Autodesk Inventor part; units mm, degrees
ref_plane "YZ Plane" through (0, 0, 0) normal (1, 0, 0) x (0, 1, 0)
ref_plane "XZ Plane" through (0, 0, 0) normal (0, 1, 0) x (-1, 0, 0)
ref_plane "XY Plane" through (0, 0, 0) normal (0, 0, 1) x (1, 0, 0)
sketch "Boceto1" plane through (0, 0, 0) normal (0, 0, 1) x (1, 0, 0)
  line L0 (-46, -14.91) -> (-46, -35.91)
  line L1 (-44.1, -31.91) -> (-2.9, -31.91)
  line L2 (-1, -35.91) -> (-1, -20.31)
  line L3 (-8.1, 6.6131) -> (-8.1, -14.91)
  line L4 (-44.6, -16.31) -> (-6.4, -16.31)
  line L5 (-2.4, -20.31) -> (-2.4, -30.01)
  line L6 (-2.9, -30.51) -> (-44.1, -30.51)
  line L7 (-44.6, -30.01) -> (-44.6, -16.31)
  arc A0 (-2.4, -20.31) -> (-6.4, -16.31) centre (-6.4, -20.31) ccw
  line L8 (-2.4, -32.41) -> (-2.4, -34.1632)
  line L9 (-3.5, -35.91) -> (-1, -35.91)
  line L10 (-9.5, -14.91) -> (-9.5, 7.7994)
  line L11 (-44.6, -32.41) -> (-44.6, -34.2323)
  line L12 (-43.5, -35.91) -> (-46, -35.91)
  line L13 (-43.5, -35.91) -> (-43.5, -35.4546)
  line L14 (-3.5, -35.91) -> (-3.5, -35.21)
  line L15 (-43.7447, -35.0247) -> (-44.3553, -34.6622)
  line L16 (-3.5, -35.21) -> (-2.6082, -34.5692)
  arc A1 (-2.9, -30.51) -> (-2.4, -30.01) centre (-2.9, -30.01) ccw
  arc A2 (-2.4, -32.41) -> (-2.9, -31.91) centre (-2.9, -32.41) ccw
  arc A3 (-2.6082, -34.5692) -> (-2.4, -34.1632) centre (-2.9, -34.1632) ccw
  arc A4 (-44.6, -30.01) -> (-44.1, -30.51) centre (-44.1, -30.01) ccw
  arc A5 (-44.1, -31.91) -> (-44.6, -32.41) centre (-44.1, -32.41) ccw
  arc A6 (-44.6, -34.2323) -> (-44.3553, -34.6622) centre (-44.1, -34.2323) ccw
  arc A7 (-43.5, -35.4546) -> (-43.7447, -35.0247) centre (-44, -35.4546) ccw
  line L17 (-9.5, 7.7994) -> (-4.75, 8.59)
  line L18 (-4.75, 8.59) -> (0, 7.7994)
  line L19 (-8.1, 6.6131) -> (-4.75, 7.1707)
  line L20 (-4.75, 7.1707) -> (-1.4, 6.6131)
  line L21 (0, 7.7994) -> (0, 0)
  line L22 (0, 0) -> (-1.4, 0)
  line L23 (-1.4, 0) -> (-1.4, 6.6131)
  line L24 (-8.1, -14.91) -> (-6.4, -14.91)
  arc A8 (-1, -20.31) -> (-6.4, -14.91) centre (-6.4, -20.31) ccw
  line L25 (-4.75, 16.5254) -> (-4.75, 0) construction
  line L26 (-38.9, 6.6131) -> (-38.9, -14.91)
  line L27 (-37.5, -14.91) -> (-37.5, 7.7994)
  line L28 (-37.5, 7.7994) -> (-42.25, 8.59)
  line L29 (-42.25, 8.59) -> (-47, 7.7994)
  line L30 (-38.9, 6.6131) -> (-42.25, 7.1707)
  line L31 (-42.25, 7.1707) -> (-45.6, 6.6131)
  line L32 (-47, 7.7994) -> (-47, 0)
  line L33 (-47, 0) -> (-45.6, 0)
  line L34 (-45.6, 0) -> (-45.6, 6.6131)
  line L35 (-42.25, 16.5254) -> (-42.25, 0) construction
  line L36 (-9.5, -14.91) -> (-37.5, -14.91)
  line L37 (-38.9, -14.91) -> (-46, -14.91)
  line L38 (-23.5, 14.1873) -> (-23.5, -36.7854) construction
  point P0 (-44.6, -34.5169)
  point P1 (-43.5, -35.17)
  dimension "d17" = 4
  dimension "d24" = 1.4
  dimension "d50" = 0.7
  dimension "d61" = 0.74
  dimension "d62" = 30.7
  dimension "d63" = 35.7
  dimension "d206" = 1.4
  dimension "d207" = 1.4
  dimension "d210" = 1.4
  dimension "d211" = 1.4
  dimension "d213" = 14.2
  dimension "d214" = 1.4
  dimension "d215" = 1.4
  dimension "d216" = 1.4
  dimension "d217" = 1.4
  dimension "d218" = 45
  dimension "d223" = 5.4
  dimension "d224" = 1.4
  dimension "d225" = 9.5
  dimension "d226" = 4.75
  dimension "d227" = 3.35
  dimension "d228" = 6.7
  dimension "d229" = 44.5
  dimension "d230" = 3.35
  dimension "d231" = 2.5
  dimension "d232" = 2.5
  dimension "d240" = 8.59
  dimension "d241" = 3.35
  dimension "d242" = 99.45
  dimension "d243" = 161.1
  dimension "d246" = 1.4
  dimension "d247" = 1.4
  dimension "d248" = 1.4
  dimension "d253" = 1.4
  dimension "d254" = 1.4
  dimension "d255" = 1.4
  dimension "d256" = 1.4
  dimension "d257" = 8.59
  dimension "d258" = 161.1
  dimension "d259" = 99.45
  dimension "d260" = 22.5
  dimension "d266" = 23.5
  dimension "d267" = 47
  dimension "d268" = 3.35
  dimension "d269" = 9.5
  dimension "d270" = 4.75
  dimension "d271" = 3.35
  dimension "d272" = 6.7
  dimension "d273" = 28
  dimension "d274" = 37.5
  dimension "d275" = 8.5
  dimension "d276" = 8.5
  dimension "d277" = 44.5
  dimension "d278" = 0.5
  dimension "d279" = 14.91
  dimension "d280" = 14.91
  dimension "d283" = 16.5254
  dimension "d284" = 0
  dimension "d285" = 14.1873
  dimension "d286" = 36.7854
  dimension "d287" = 16.5254
  dimension "d288" = 0
extrude "Extrusión1" add sketch "Boceto1" against normal blind 1400
ref_plane "Plano de trabajo1" through (0, 0, -700) normal (0, 0, -1) x (-1, 0, 0)
sketch "Boceto2" plane through (0, 0, 0) normal (1, 0, 0) x (0, 1, 0)
  line L0 (-35.91, 0) -> (-20.31, 0)
  line L1 (-35.91, 0) -> (-35.91, -1400)
  line L2 (-20.31, -1400) -> (-35.91, -1400)
  line L3 (-20.31, 0) -> (-20.31, -1400)
  line L4 (-20.31, 0) -> (-14.91, 0)
  line L5 (-20.31, 0) -> (-20.31, -1400)
  line L6 (-14.91, -1400) -> (-20.31, -1400)
  line L7 (-14.91, 0) -> (-14.91, -1400)
  line L8 (-14.91, 0) -> (6.6131, 0)
  line L9 (-14.91, 0) -> (-14.91, -1400)
  line L10 (6.6131, -1400) -> (-14.91, -1400)
  line L11 (6.6131, 0) -> (6.6131, -1400)
  line L12 (0, 0) -> (7.7994, 0)
  line L13 (0, 0) -> (0, -1400)
  line L14 (7.7994, -1400) -> (0, -1400)
  line L15 (7.7994, 0) -> (7.7994, -1400)
  line L16 (7.7994, 0) -> (8.59, 0)
  line L17 (7.7994, 0) -> (7.7994, -1400)
  line L18 (8.59, -1400) -> (7.7994, -1400)
  line L19 (8.59, 0) -> (8.59, -1400)
  line L20 (-35.91, 0) -> (8.59, -44.5)
  line L21 (8.59, 0) -> (8.59, -44.5)
  line L22 (8.59, 0) -> (-35.91, 0)
  dimension "d291" = 45
extrude "Extrusión2" cut sketch "Boceto2" against normal through all contours L0 L3 L20 | L4 L7 L20 L3 | L8 L13 L20 L7 | L8 L11 L20 L13 | L12 L15 L20 L11 | L16 L19 L20 L15
mirror "Simetría1" about plane through (0, 0, -700) normal (0, 0, -1) of "Extrusión2"
properties part number "SP40-09 MARCO CORREDERA 1400 MM" material "Aluminio"
Can you work these out from the model? Positions are in its coordinate system, mm. A direction names the side the tool comes from. Coordinates: 2 decimals unless noted, no trailing zeros. Answer as a JSON object with one key per item and string values.
1) For P1, Ø23, axis at y = -28.5, z = -955.5, coming from the -X side; P2, Ø2, axis at x = -34.5, y = -30.5, coming from the +Z side; P3, Ø11, axis at y = -9, z = -426, coming from the -X side, each with a flat end and sliding along its axis, tell me the tip position at first contact or that it passes through.
Results:
{"P1": "stops at x = -46", "P2": "stops at z = -4.41", "P3": "stops at x = -38.9"}
2) If I drill on line 1 (X direction, y = 1, z = -144); line 2 (X direction, y = -3, z = -236); line 3 (X direction, y = -26.5, z = -1110), over which ranges is the centre line in solid material (lowest first)?
Results:
{"line 1": "x = -47 to -45.6, -38.9 to -37.5, -9.5 to -8.1, -1.4 to 0", "line 2": "x = -38.9 to -37.5, -9.5 to -8.1", "line 3": "x = -46 to -44.6, -2.4 to -1"}
3) Thinking about a two-plate mould opening in Y: for faces 4 (the face through (-9.5, -4, -690)), 5 (the face through (-21.65, -15.41, -20.5)), 6 (the face through (-8.1, -4, -690)), which applies, pulls with the +Y half, pulls with the -Y half, needs draft (parallel to the pull), parting line crosses it, or undercut?
Results:
{"face 4": "needs draft", "face 5": "pulls with the +Y half", "face 6": "undercut"}
4) For faces 1 (the face through (-21.65, -15.2, -1379.29)), 2 (the face through (-37.5, -4, -690)), 3 (the face through (-26, -16.31, -690)), which set-ups out of +Z, -Z, +X, -X, +Y, -Y let a thin tool reach every point of the face, with its end or its side?
Results:
{"face 1": "-Z, +X, -X, +Y", "face 2": "+Z, -Z, +Y", "face 3": "+Z, -Z"}
